Autodesk Inventor part; units mm, degrees
ref_plane "YZ Plane" through (0, 0, 0) normal (1, 0, 0) x (0, 1, 0)
ref_plane "XZ Plane" through (0, 0, 0) normal (0, 1, 0) x (-1, 0, 0)
ref_plane "XY Plane" through (0, 0, 0) normal (0, 0, 1) x (1, 0, 0)
sketch "Sketch1" plane through (0, 0, 0) normal (0, 1, 0) x (-1, 0, 0)
  line L0 (0, 329.241) -> (0, -329.241) construction
  line L1 (203.5937, 0) -> (-203.5937, 0) construction
  arc A0 (-441.1, 0) -> (250, -363.4133) centre (0, 0) ccw
  line L2 (-441.1, 0) -> (-441.1, 400)
  line L3 (-441.1, 400) -> (-500, 400)
  line L4 (-500, 400) -> (-500, -500)
  line L5 (-500, -500) -> (250, -500)
  line L6 (250, -500) -> (250, -363.4133)
  dimension "d0" = 500
  dimension "d1" = 400
  dimension "d2" = 500
  dimension "d3" = 441.1
  dimension "d4" = 750
extrude "Extrusion1" add sketch "Sketch1" along normal blind 5
properties part number "boundaryV1"
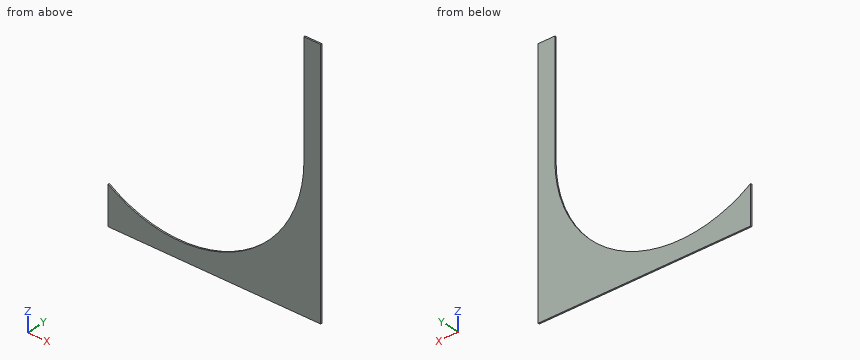
Read the model definition and answer for the solid it produces. Units are mm, in the model's axes. Give positions to 0.01 mm unless a question says otherwise; leave off trailing zeros. Write each loop counter-clockwise with the first axis right and the second up, starting at its lowest first coordinate (ties: lowest second). Pieces come first, ordered by that corner, then holes. Notation, with made-up numbers: (10, 57) -> (68, 57) arc R11 cw to (68, 64) -> close; hole circle Ø1 at (66.5, 19). An arc over 180 degrees is marked (long way). Answer as a JSON object with one key per item and string values. Group by question number.
1) Find section D-D (x = -4.5). Write down the section's boundary in (y, z), and give its area (3 significant figures).
2) Find section C-C (z = 64.5). Write down the section's boundary in (x, y).
3) Each of these flat-tipped pins is pushed along its axis until it touches: P1, Ø1.5, axis at y = 4, z = -360.5, coming from the -X side; P2, Ø1.5, axis at y = 1.5, z = 203, coming from the -X side. Where does it stop, or does it pass through?
4) Consider L1, parallel to X at y = 1.25, z = 355; L2, parallel to Z at x = 9, y = 2.55; L3, parallel to X at y = 2.35, z = -364.5. Determine where each line is inside the solid, lowest interval first. Write a range as from..to.
5) Find section A-A (z = -405.5). Write down the section's boundary in (x, y).
6) Find section B-B (y = 3.85). Write down the section's boundary in (x, z), and give its area (3 significant figures).
Values follow:
{
 "1": {"outline": "(0, -500) -> (5, -500) -> (5, -441.08) -> (0, -441.08) -> close", "area": "295 mm2"},
 "2": {"outline": "(441.1, 0) -> (500, 0) -> (500, 5) -> (441.1, 5) -> close"},
 "3": {"P1": "stops at x = 253.12", "P2": "stops at x = 441.1"},
 "4": {"L1": "x = 441.1..500", "L2": "z = -500..-441.01", "L3": "x = -250..-248.41, 248.41..500"},
 "5": {"outline": "(-250, 0) -> (-173.61, 0) -> (-173.61, 5) -> (-250, 5) -> close; (173.61, 0) -> (500, 0) -> (500, 5) -> (173.61, 5) -> close"},
 "6": {"outline": "(-250, -500) -> (500, -500) -> (500, 400) -> (441.1, 400) -> (441.1, 0) arc R441.1 cw to (-250, -363.41) -> close", "area": "142,000 mm2"}
}
